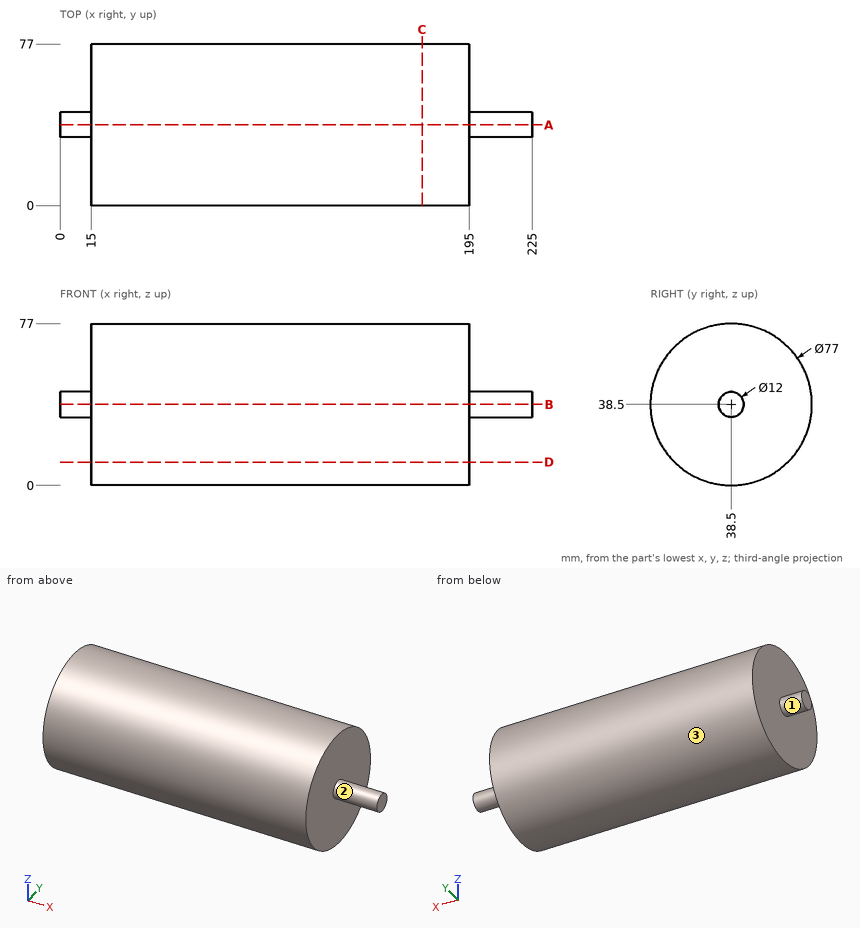
Part print with two shaded views. Sizes in mm from the minimum x, y, z corner. A direction names the side the tool comes from. Round coordinates to 2 decimals unless told otherwise and drop trailing zeros. Order: outer loops, then holes, each group sorted by start corner. A loop starts at its lowest first (then second) coordinate and runs counter-clockwise, first axis right, second up.
(1) 3-axis set-ups, long thin cutter, end or side, ignore diameter. For the marked faces 1, 2 and 3: which of +Z, -Z, +X, -X, +Y, -Y reach the whole face in a straight line?
(2) Band-saw the part on C-C (x = 172.5). List the corners of the cut face in (y, z).
(3) Pin check, flat tips, straight feed: pin 1 (5 mm diameter, centred on y = 49, z = 38, fed in from -X); pin 2 (5 mm diameter, centred on x = 186, y = 20.5, fed in from -Z); pin 3 (10 mm diameter, centred on x = 85.5, y = 32.5, fed in from -Z). Stop position of each tip, or through.
(4) Band-saw the part on A-A (y = 38.5). List the corners of the cut face in (x, z).
(5) Band-saw the part on D-D (z = 11). List the corners of the cut face in (x, y), then the cut area to 3 significant figures.
(6) Drill centre lines: line 1 (X direction, y = 33, z = 13); line 2 (Y direction, x = 51, z = 61); line 3 (Y direction, x = 158, z = 8.5). Where is each one in solid material? Low to high.
Verdict:
1. face 1: -X
1. face 2: +X
1. face 3: +X, -X
2. outline: circle Ø77 at (38.5, 38.5)
3. pin 1: stops at x = 15
3. pin 2: stops at z = 3.26
3. pin 3: stops at z = 0.01
4. outline: (0, 32.5) - (15, 32.5) - (15, 0) - (195, 0) - (195, 32.5) - (225, 32.5) - (225, 44.5) - (195, 44.5) - (195, 77) - (15, 77) - (15, 44.5) - (0, 44.5) - close
5. outline: (15, 11.56) - (195, 11.56) - (195, 65.44) - (15, 65.44) - close
5. area: 9,700 mm2
6. line 1: x = 15 to 195
6. line 2: y = 7.26 to 69.74
6. line 3: y = 14.37 to 62.63
